CAD build for the part. Positions are in the model's coordinates, mm. A direction names the side the tool comes from. Round coordinates to 2 decimals unless told otherwise and drop trailing zeros. Loops run counter-clockwise (first coordinate to the right, second up) from the corner with the lowest first, then second, coordinate; pieces in that order, holes last. Notation, with made-up numbers: (65.25, -30) - (71.25, -30) arc R25 cw to (71.25, -14) - close; hole circle Ø2 at (29.25, 58). An arc over 180 degrees is marked (long way). Use one line per item in the form item = value.
from build123d import *

# Parameters (mm, degrees)
F0_W     = 85.31113
F0_H     = 40.683054
F1_DEPTH = 12.7
F2_R     = 5.08
F3_T     = -2.54
F5_DEPTH = 2.54


with BuildPart() as f1:
    # F0 (on Top) → F1 (new body, symmetric)
    with BuildSketch(Plane.XY):
        Rectangle(F0_W, F0_H)
    extrude(amount=F1_DEPTH, both=True)

    # F2
    f2_edges = [f1.edges().sort_by_distance(p)[0] for p in [
        (42.655565, -20.341527, 0),
        (42.655565, 20.341527, 0),
        (-42.655565, -20.341527, 0),
        (-42.655565, 20.341527, 0),
    ]]
    fillet(f2_edges, radius=F2_R)

    # F3
    f3_openings = [f1.faces().sort_by_distance(p)[0] for p in [
        (0, 0, 12.7),
    ]]
    offset(amount=F3_T, openings=f3_openings)

    # F4 (on face) → F5 (cut, through all)
    with BuildSketch(Plane.XY.offset(-10.16)):
        Polygon((-7.482303, 5.966937), (-9.330279, -2.129575), (-4.152365, -8.622474), (4.152365, -8.622474), (9.330279, -2.129575), (7.482303, 5.966937), (0, 9.570225), align=None)
    extrude(amount=-F5_DEPTH, mode=Mode.SUBTRACT)


solid = f1.part
1) Slice it at D-D (y = 7.5). Write the cut outline in (x, z).
Report:
outline = (-42.66, -12.7) - (-4.3, -12.7) - (-4.3, -10.16) - (-40.12, -10.16) - (-40.12, 12.7) - (-42.66, 12.7) - close; (4.3, -12.7) - (42.66, -12.7) - (42.66, 12.7) - (40.12, 12.7) - (40.12, -10.16) - (4.3, -10.16) - close
2) Flat gauge pin, fed straight in: pin 1 (1 mm diameter, centred on x = -16.5, y = -15.5, fed in from +Z). Where does the tip first touch, or does it go through?
Report:
pin_1 = -10.16
3) Slice it at A-A (x = -1). Write the cut outline in (y, z), plus the area to 3 significant figures.
Report:
outline = (-20.34, -12.7) - (-8.62, -12.7) - (-8.62, -10.16) - (-17.8, -10.16) - (-17.8, 12.7) - (-20.34, 12.7) - close; (9.09, -12.7) - (20.34, -12.7) - (20.34, 12.7) - (17.8, 12.7) - (17.8, -10.16) - (9.09, -10.16) - close
area = 174 mm^2
4) Slice it at C-C (x = -32.5). Write the cut outline in (y, z).
Report:
outline = (-20.34, -12.7) - (20.34, -12.7) - (20.34, 12.7) - (17.8, 12.7) - (17.8, -10.16) - (-17.8, -10.16) - (-17.8, 12.7) - (-20.34, 12.7) - close
5) Two-plate mould, pull along X, no slides. Class faces 1 (the cylindrical face through (41.21, 18.81, -0.18)), 2 (the flat face through (-1, -17.802, 1)), 3 (the cylindrical face through (-41.21, -18.81, 0.18)): +X half, -X half, draft (parallel to the pull), parting line (faces both ways), or undercut.
Report:
face_1 = +X half
face_2 = undercut
face_3 = -X half
6) Drill centre lines: probe 1 along Y at (x, z) = (11.5, 7.5); probe 2 along X at (y, z) = (-9, -2); probe 3 along Z at (x, y) = (8.5, -17). Where is each one in solid material? Low to high.
Report:
probe_1 = -20.34 to -17.8, 17.8 to 20.34
probe_2 = -42.66 to -40.12, 40.12 to 42.66
probe_3 = -12.7 to -10.16
7) Slice it at B-B (z = -1). Write the cut outline in (x, y).
Report:
outline = (-42.66, -15.26) arc R5.08 ccw to (-37.58, -20.34) - (37.58, -20.34) arc R5.08 ccw to (42.66, -15.26) - (42.66, 15.26) arc R5.08 ccw to (37.58, 20.34) - (-37.58, 20.34) arc R5.08 ccw to (-42.66, 15.26) - close; hole (-40.12, -15.26) arc R2.54 ccw to (-37.58, -17.8) - (37.58, -17.8) arc R2.54 ccw to (40.12, -15.26) - (40.12, 15.26) arc R2.54 ccw to (37.58, 17.8) - (-37.58, 17.8) arc R2.54 ccw to (-40.12, 15.26) - close
8) Tool access for faces 4 (the flat face through (0, -8.622, -11)), 5 (the flat face through (-3, -18, 12.7)), 6 (the cylindrical face through (-39.39, -17.04, 1.43)): list every direction of +Z, -Z, +X, -X, +Y, -Y with a clear straight run to the whole face (end or side of a thin tool).
Report:
face_4 = +Z, -Z
face_5 = +Z, +X, -X, +Y, -Y
face_6 = +Z
